Autodesk Inventor part; units mm, degrees
ref_plane "YZ Plane" through (0, 0, 0) normal (1, 0, 0) x (0, 1, 0)
ref_plane "XZ Plane" through (0, 0, 0) normal (0, 1, 0) x (-1, 0, 0)
ref_plane "XY Plane" through (0, 0, 0) normal (0, 0, 1) x (1, 0, 0)
sketch "スケッチ1" plane through (0, 0, 0) normal (0, 0, 1) x (1, 0, 0)
  circle A0 centre (0, 0) radius 4
  circle A1 centre (0, 0) radius 2
  dimension "d0" = 8
  dimension "d1" = 4
extrude "押し出し1" add sketch "スケッチ1" along normal blind 20
fillet "フィレット1" radius 0.3 2 edges at (-4, 0, 20) (-4, 0, 0)
thread "ねじ1"
extrude "押し出し2" add sketch "スケッチ1" along normal blind 15 contours A1
extrude "押し出し3" cut sketch "スケッチ1" along normal blind 6 contours A1
thread "ねじ2"
properties part number "スペーサーM4L20アルミ" material "アルミニウム 2014-T4"
Check sheet for the modelled part. Datum: model origin and axes. Units: mm. A direction names the side the tool comes from. Give positions to 0.01 mm unless a question says otherwise; leave off trailing zeros. Loops run counter-clockwise (first coordinate to the right, second up) from the corner with the lowest first, then second, coordinate; pieces in that order, holes last. Notation, with made-up numbers: M 0,21.5 L 12,21.5 A28 ccw 12,56.5 Z; hole C -25,48.5 d2. An arc over 180 degrees is marked long. Return JSON: item names as keys, results as strings. Group by question number.
1. Thickness scan on L1, parallel to Y at x = 0, z = 18.25; L2, parallel to X at y = 1.5, z = 3.5; L3, parallel to X at y = -0.5, z = 2.25. Record the ranges inside material, lowest first.
2. Cross-section at C-C on z = 4.5. Record the boundary of the cut face in (x, y).
3. Tool access check on faces 4 (the flat face through (0, 0, 15)), 5 (the cylindrical face through (0, 2, 3)), 6 (the flat face through (2, -2, 0)). Record the directions out of +Z, -Z, +X, -X, +Y, -Y that give a thin tool (end or side, any length) a straight path to the whole face; none if there is none.
4. Cross-section at A-A on x = 0. Record the boundary of the cut face in (y, z), plus the area to 3 significant figures.
5. Mould release check, pull along Y, two halves, no side actions. Record for faces 1 (the flat face through (2, -2, 20)), 2 (the flat face through (0, 0, 6)), 3 (the cylindrical face through (-0.867, 3.905, 9.864)): released by +Y, released by -Y, zero draft, split by the parting line, or undercut.
6. Go/stop test with flat-tipped pins: pin 1 (1.5 mm diameter, centred on x = 2.5, z = 14, fed in from +Y); pin 2 (3 mm diameter, centred on x = 0, y = 0, fed in from -Z). Record where each tip stops, or that it passes through.
7. Cross-section at D-D on z = 7.5. Record the boundary of the cut face in (x, y).
Return value:
{
 "1": {"L1": "-4 to -2, 2 to 4", "L2": "-3.71 to -1.32, 1.32 to 3.71", "L3": "-3.97 to -1.94, 1.94 to 3.97"},
 "2": {"outline": "C 0,0 d8; hole C 0,0 d4"},
 "3": {"face 4": "+Z", "face 5": "-Z", "face 6": "-Z, +X, -X, +Y, -Y"},
 "4": {"outline": "M -4,0.3 A0.3 ccw -3.7,0 L -2,0 L -2,6 L 2,6 L 2,0 L 3.7,0 A0.3 ccw 4,0.3 L 4,19.7 A0.3 ccw 3.7,20 L 2,20 L 2,15 L -2,15 L -2,20 L -3.7,20 A0.3 ccw -4,19.7 Z", "area": "116 mm^2"},
 "5": {"face 1": "zero draft", "face 2": "undercut", "face 3": "split by the parting line"},
 "6": {"pin 1": "y = 3.6", "pin 2": "z = 6"},
 "7": {"outline": "C 0,0 d8"}
}
